Here's how the part is built. I have some questions about the finished solid (model axes, mm). Face numbers are marked on the shaded views. A direction names the side the tool comes from. Give positions to 0.01 mm unless a question says otherwise; leave off trailing zeros. Write each loop counter-clockwise with the first axis right and the second up, starting at its lowest first coordinate (ties: lowest second). Pieces come first, ordered by that corner, then holes. Notation, with made-up numbers: (4.25, 63) -> (19.25, 63) arc R15 cw to (19.25, 74) -> close; hole circle Ø7 at (42, 0.5). An arc over 180 degrees is marked (long way). Return JSON: item names as keys, results as strings.
from build123d import *

# Parameters (mm, degrees)
F1_DEPTH = 33
F2_R     = 1.1
F2_W     = 6.2774603256
F2_H     = 1.5
F3_DEPTH = 42.501
F5_DEPTH = 15
F7_DEPTH = 42.501
F8_R     = 4
F8_R_2   = 1.1
F9_DEPTH = 1.5


with BuildPart() as f1:
    # F0 (on Front) → F1 (new body)
    with BuildSketch(Plane.XZ):
        Polygon((0, 26.5), (0, 0), (1.5, 0), (1.5, 25), (41, 25), (41, 0), (42.5, 0), (42.5, 26.5), align=None)
    extrude(amount=F1_DEPTH)

    # F2 (on face) → F3 (cut, through all)
    with BuildSketch(Plane(origin=(0, 0, 0), x_dir=(0, -1, 0), z_dir=(-1, 0, 0))):
        with BuildLine():
            Line((20.5, 0), (20.5, 2))
            ThreePointArc((20.5, 2), (16.5, 6), (12.5, 2))
            Line((12.5, 2), (12.5, 0))
            Line((12.5, 0), (20.5, 0))
        make_face()
        with Locations((22.7225396744, 2)):
            Circle(F2_R)
        with Locations((20.9, 6.4)):
            Circle(F2_R)
        with Locations((16.5, 8.2225396744)):
            Circle(F2_R)
        with Locations((12.1, 6.4)):
            Circle(F2_R)
        with Locations((10.2774603256, 2)):
            Circle(F2_R)
        Polygon((0, 0), (6.2774603256, 0), (0, 25), align=None)
        Polygon((0, 25), (6.2774603256, 0), (6.2774603256, 25), align=None)
        with Locations((3.1387301628, 25.75)):
            Rectangle(F2_W, F2_H)
        Polygon((26.7225396744, 0), (33, 0), (33, 25), align=None)
        Polygon((26.7225396744, 0), (33, 25), (26.7225396744, 25), align=None)
        with Locations((29.8612698372, 25.75)):
            Rectangle(F2_W, F2_H)
    extrude(amount=-F3_DEPTH, mode=Mode.SUBTRACT)

    # F4 (on face) → F5 (join)
    with BuildSketch(Plane.XZ.offset(26.7225396744)):
        Polygon((1.5, 0), (1.5, 25), (41, 25), (41, 0), (42.5, 0), (42.5, 26.5), (0, 26.5), (0, 0), align=None)
    extrude(amount=F5_DEPTH)

    # F6 (on face) → F7 (cut, through all)
    with BuildSketch(Plane.YZ.offset(42.5)):
        Polygon((-26.7225396744, 0), (-41.7225396744, 25), (-41.7225396744, 0), align=None)
    extrude(amount=-F7_DEPTH, mode=Mode.SUBTRACT)

    # F8 (on face) → F9 (cut, through all)
    with BuildSketch(Plane.XY.offset(26.5)):
        with Locations((21.25, -31.7225396744)):
            Circle(F8_R)
        with Locations((21.25, -37.7225396744)):
            Circle(F8_R_2)
        with Locations((25.4926406871, -35.9651803616)):
            Circle(F8_R_2)
        with Locations((27.25, -31.7225396744)):
            Circle(F8_R_2)
        with Locations((25.4926406871, -27.4798989873)):
            Circle(F8_R_2)
        with Locations((21.25, -25.7225396744)):
            Circle(F8_R_2)
        with Locations((17.0073593129, -27.4798989873)):
            Circle(F8_R_2)
        with Locations((15.25, -31.7225396744)):
            Circle(F8_R_2)
        with Locations((17.0073593129, -35.9651803616)):
            Circle(F8_R_2)
    extrude(amount=-F9_DEPTH, mode=Mode.SUBTRACT)


solid = f1.part
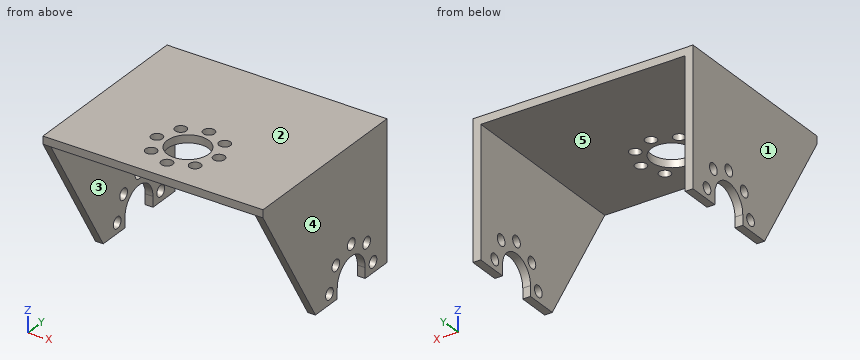
1. For pin 1 Ø3 at (x, y) = (25.49, -27.48) entering from -Z; pin 2 Ø0.8 at (x, z) = (41.5, 1) entering from -Y, each with a flat end and sliding along its axis, tell me the tip position at first contact or that it passes through.
Taken from the geometry:
{"pin 1": "stops at z = 25", "pin 2": "stops at y = -27.56"}
2. Suppose I cut it at A-A, the plane x = 15.25. List the corners of the cut face in (y, z) for me, and give its area (3 significant figures).
Taken from the geometry:
{"outline": "(-41.72, 25) -> (-32.82, 25) -> (-32.82, 26.5) -> (-41.72, 26.5) -> close; (-30.62, 25) -> (-6.28, 25) -> (-6.28, 26.5) -> (-30.62, 26.5) -> close", "area": "49.9 mm²"}
3. Suppose I cut it at B-B, the plane y = -16.5. List the corners of the cut face in (x, z) for me, and give its area (3 significant figures).
Taken from the geometry:
{"outline": "(0, 6) -> (1.5, 6) -> (1.5, 7.12) -> (0, 7.12) -> close; (0, 9.32) -> (1.5, 9.32) -> (1.5, 25) -> (41, 25) -> (41, 9.32) -> (42.5, 9.32) -> (42.5, 26.5) -> (0, 26.5) -> close; (41, 6) -> (42.5, 6) -> (42.5, 7.12) -> (41, 7.12) -> close", "area": "114 mm²"}
4. If I drill on line 1 (Y direction, x = 27.25, z = 26.15); line 2 (X direction, y = -21, z = 24.5); line 3 (Z direction, x = 39.5, y = -39.5), over which ranges is the centre line in solid material (lowest first)? Write a range as [from, to].
Taken from the geometry:
{"line 1": "y = [-41.72, -32.82], [-30.62, -6.28]", "line 2": "x = [0, 1.5], [41, 42.5]", "line 3": "z = [25, 26.5]"}
5. Suppose I cut it at C-C, the plane x = 21.25. List the corners of the cut face in (y, z) for me, and give its area (3 significant figures).
Taken from the geometry:
{"outline": "(-41.72, 25) -> (-38.82, 25) -> (-38.82, 26.5) -> (-41.72, 26.5) -> close; (-36.62, 25) -> (-35.72, 25) -> (-35.72, 26.5) -> (-36.62, 26.5) -> close; (-27.72, 25) -> (-26.82, 25) -> (-26.82, 26.5) -> (-27.72, 26.5) -> close; (-24.62, 25) -> (-6.28, 25) -> (-6.28, 26.5) -> (-24.62, 26.5) -> close", "area": "34.6 mm²"}
6. Which directions (+Z, -Z, +X, -X, +Y, -Y) give clear straight access to the entire face, cutting with the end or side of a thin tool? Please do the marked faces 4 and 5.
Taken from the geometry:
{"face 4": "+Z, -Z, +X, +Y, -Y", "face 5": "-Z, +Y, -Y"}
7. If we mould it in two halves opening along X, with no side actions, what happens to the marked faces 1, 2 and 3? For each: released by +X, released by -X, zero draft, split by the parting line, or undercut.
Taken from the geometry:
{"face 1": "released by -X", "face 2": "zero draft", "face 3": "undercut"}
8. Suppose I cut it at D-D, the plane z = 22. List the corners of the cut face in (x, y) for me.
Taken from the geometry:
{"outline": "(0, -39.92) -> (1.5, -39.92) -> (1.5, -6.28) -> (0, -6.28) -> close; (41, -39.92) -> (42.5, -39.92) -> (42.5, -6.28) -> (41, -6.28) -> close"}
